```python
from build123d import *

# Parameters (mm, degrees)
SKETCH1_R             = 2.5
BOSS_EXTRUDE1_DEPTH   = 25
BOSS_EXTRUDE1_2_DEPTH = 25
BOSS_EXTRUDE2_DEPTH   = 38
SKETCH1_4_R           = 2.5
BOSS_EXTRUDE3_DEPTH   = 23
SKETCH1_5_R           = 3.4
SKETCH1_5_R_2         = 1
BOSS_EXTRUDE4_DEPTH   = 20


with BuildPart() as part:
    # Sketch1 → Boss-Extrude1 (new body)
    with BuildSketch(Plane(origin=(0, 0, 0), x_dir=(1, 0, 0), z_dir=(0, 1, 0))):
        with BuildLine():
            ThreePointArc((-3.4, 0), (0, 3.4), (3.4, 0))
            Line((3.4, 0), (4.85054735, 8.226462813))
            ThreePointArc((4.85054735, 8.226462813), (0, 9.55), (-4.85054735, 8.226462813))
            Line((-4.85054735, 8.226462813), (-3.4, 0))
        make_face()
        with Locations(Location((0, 6.475, 0), (0, 0, 270))):
            Circle(SKETCH1_R, mode=Mode.SUBTRACT)
    extrude(amount=BOSS_EXTRUDE1_DEPTH)



with BuildPart() as body_2:
    # Sketch1 → Boss-Extrude1 2 (new body)
    with BuildSketch(Plane(origin=(0, 0, 0), x_dir=(1, 0, 0), z_dir=(0, 1, 0))):
        with BuildLine():
            Line((4.85054735, -8.226462813), (3.4, 0))
            ThreePointArc((3.4, 0), (0, -3.4), (-3.4, 0))
            Line((-3.4, 0), (-4.85054735, -8.226462813))
            ThreePointArc((-4.85054735, -8.226462813), (0, -9.55), (4.85054735, -8.226462813))
        make_face()
        with Locations(Location((0, -6.475, 0), (0, 0, 270))):
            Circle(SKETCH1_R, mode=Mode.SUBTRACT)
    extrude(amount=BOSS_EXTRUDE1_2_DEPTH)


with BuildPart() as part_1:
    add(part.part)

    add(body_2.part)  # Boss-Extrude2 merges body 2
    # Sketch1<3> → Boss-Extrude2 (add)
    with BuildSketch(Plane(origin=(0, 0, 0), x_dir=(1, 0, 0), z_dir=(0, 1, 0))):
        with BuildLine():
            Line((4.85054735, 8.226462813), (3.4, 0))
            Line((3.4, 0), (4.85054735, -8.226462813))
            ThreePointArc((4.85054735, -8.226462813), (8.292322569, -4.737075723), (9.55, 0))
            ThreePointArc((9.55, 0), (8.292322569, 4.737075723), (4.85054735, 8.226462813))
        make_face()
        with BuildLine():
            Line((-4.85054735, -8.226462813), (-3.4, 0))
            Line((-3.4, 0), (-4.85054735, 8.226462813))
            ThreePointArc((-4.85054735, 8.226462813), (-9.55, 0), (-4.85054735, -8.226462813))
        make_face()
    extrude(amount=BOSS_EXTRUDE2_DEPTH)

    # Sketch1<4> → Boss-Extrude3 (add)
    with BuildSketch(Plane(origin=(0, 0, 0), x_dir=(1, 0, 0), z_dir=(0, 1, 0))):
        with Locations(Location((0, -6.475, 0), (0, 0, 270))):
            Circle(SKETCH1_4_R)
        with Locations(Location((0, 6.475, 0), (0, 0, 270))):
            Circle(SKETCH1_4_R)
    extrude(amount=BOSS_EXTRUDE3_DEPTH)

    # Sketch1<5> → Boss-Extrude4 (add)
    with BuildSketch(Plane(origin=(0, 0, 0), x_dir=(1, 0, 0), z_dir=(0, 1, 0))):
        Circle(SKETCH1_5_R)
        with Locations(Location((0, 0, 0), (0, 0, 270))):
            Circle(SKETCH1_5_R_2, mode=Mode.SUBTRACT)
    extrude(amount=BOSS_EXTRUDE4_DEPTH)


solid = part_1.part
```
Can you work these out from the model? Positions are in its coordinate system, mm. A direction names the side the tool comes from. Coordinates: 2 decimals unless noted, no trailing zeros. Order: outer loops, then holes, each group sorted by start corner. A loop starts at its lowest first (then second) coordinate and runs counter-clockwise, first axis right, second up.
1. Thinking about a two-plate mould opening in X: for faces 1 (the face through (-0.1, 25, -3.8)), 2 (the face through (6, 38, 0)), which applies, +X half, -X half, draft (parallel to the pull), parting line (faces both ways), or undercut?
2. I need wall thicknesses on line 1 (Y direction, x = -3.5, z = 2.25); line 2 (X direction, y = 31, z = 3); line 3 (Y direction, x = -2, z = -5.25). Which ranges of each line are inside material? Lowest first, please.
3. For faces 3 (the face through (-1, 10, 0)), 4 (the face through (-7, 38, 0)), 5 (the face through (-0.1, 25, 3.6)), 6 (the face through (-4.115, 31.409, -4.056)), 7 (the face through (0.74, 22.46, 3.32)), which set-ups out of +Z, -Z, +X, -X, +Y, -Y let a thin tool reach every point of the face, with its end or its side?
4. If we section it at A-A (x = 0): Please give me the cut outline in (y, z) (3 decimals), then the cut area to 4 significant figures.
5. If we section it at B-B (y = 35.5): Please give me the cut outline in (x, z).
6. I'm going to push flat-ended pins straight in: pin 1 (4 mm diameter, centred on x = 0, z = 6.475, fed in from +Y); pin 2 (5 mm diameter, centred on x = -0.5, z = -4, fed in from +Y); pin 3 (3 mm diameter, centred on x = -3.5, y = 29, fed in from +Z). Where does each tip first touch, or does it pass through?
7. If we section it at D-D (z = 2): Please give me the cut outline in (x, y).
8. If we section it at C-C (y = 6.5): Please give me the cut outline in (x, z), then the cut area to 3 significant figures.
Entries:
1. face 1: undercut
1. face 2: draft
2. line 1: y = 0 to 25
2. line 2: x = -9.07 to -3.93, 3.93 to 9.07
2. line 3: y = 0 to 23
3. face 3: +Y, -Y
3. face 4: +Z, -Z, +X, -X, +Y
3. face 5: +Z, +Y
3. face 6: -Z, +Y
3. face 7: +Y
4. outline: (0, -9.55) - (25, -9.55) - (25, -8.975) - (23, -8.975) - (23, -3.975) - (25, -3.975) - (25, -3.4) - (20, -3.4) - (20, -1) - (0, -1) - close; (0, 1) - (20, 1) - (20, 3.4) - (25, 3.4) - (25, 3.975) - (23, 3.975) - (23, 8.975) - (25, 8.975) - (25, 9.55) - (0, 9.55) - close
4. area: 383.5 mm2
5. outline: (-4.85, -8.23) - (-3.4, 0) - (-4.85, 8.23) arc R9.55 ccw to start; (3.4, 0) - (4.85, -8.23) arc R9.55 ccw to (4.85, 8.23) - close
6. pin 1: stops at y = 23
6. pin 2: stops at y = 25
6. pin 3: stops at z = 8.23
7. outline: (-9.34, 0) - (9.34, 0) - (9.34, 38) - (3.75, 38) - (3.75, 25) - (2.75, 25) - (2.75, 20) - (-2.75, 20) - (-2.75, 25) - (-3.75, 25) - (-3.75, 38) - (-9.34, 38) - close
8. outline: circle Ø19.1 at (0, 0); hole circle Ø2 at (0, 0)
8. area: 283 mm2
